```python
from build123d import *

# Parameters (mm, degrees)
F0_R     = 46.99
F0_R_2   = 46.5836
F1_DEPTH = 9.9314
F2_W     = 5.08
F2_H     = 12.7
F3_DEPTH = 76.2
F4_W     = 5.08
F4_H     = 12.7
F5_DEPTH = 76.2


with BuildPart() as f1:
    # F0 (on Top) → F1 (new body)
    with BuildSketch(Plane.XY):
        Circle(F0_R)
        Circle(F0_R_2, mode=Mode.SUBTRACT)
    extrude(amount=F1_DEPTH)

    # F2 (on Right) → F3 (cut, symmetric)
    with BuildSketch(Plane.YZ):
        with Locations((0, 7.4041)):
            Rectangle(F2_W, F2_H)
    extrude(amount=F3_DEPTH, both=True, mode=Mode.SUBTRACT)

    # F4 (on Front) → F5 (cut, symmetric)
    with BuildSketch(Plane.XZ):
        with Locations((0, 7.4041)):
            Rectangle(F4_W, F4_H)
    extrude(amount=F5_DEPTH, both=True, mode=Mode.SUBTRACT)


solid = f1.part
```
The model under review builds one solid part; all positions refer to its coordinate system, in mm. Give positions to 0.01 mm unless a question says otherwise; leave off trailing zeros. Write each loop counter-clockwise with the first axis right and the second up, starting at its lowest first coordinate (ties: lowest second). Pieces come first, ordered by that corner, then holes. Notation, with made-up numbers: M 56,51.25 L 103,51.25 A22 ccw 103,69.25 Z; hole C 26.25,-28.5 d11. An arc over 180 degrees is marked long. Write item = value, one per line. Start each with the question number.
Q1. Clearance check with flat-ended pins moving along their axes: pin 1 (4 mm diameter, centred on x = -8.5, z = 5, fed in from -Y); pin 2 (4 mm diameter, centred on x = -33, z = 4.5, fed in from -Y); pin 3 (0.5 mm diameter, centred on x = 0, y = 47, fed in from +Z). State where each tip first meets the part, or that it passes through.
Q2. Mouldability with a two-part tool opening along X and no side actions: class faces 1 (the face through (44.432, 13.992, 4.896)), 2 (the face through (43.407, -17.997, 4.896)), 3 (the face through (-33.1, 33.1, 9.931)) as released by +X, released by -X, zero draft, split by the parting line, or undercut.
Q3. We need section A-A (y = 0). State the section outline as (x, z) points.
Q4. We need section C-C (z = 2.25). State the section outline as (x, y) points, plus the area to 3 significant figures.
Q5. For line 1 (Y direction, x = 25.5, z = 9); line 2 (X direction, y = 16, z = 8.25); line 3 (Y direction, x = 22, z = 3), list the stretches that pass through material, from the lowest coordinate up.
Result set:
q1.pin_1 = -46.54
q1.pin_2 = -35.31
q1.pin_3 = 1.05
q2.face_1 = undercut
q2.face_2 = split by the parting line
q2.face_3 = zero draft
q3.outline = M -46.99,0 L -46.58,0 L -46.58,1.05 L -46.99,1.05 Z; M 46.58,0 L 46.99,0 L 46.99,1.05 L 46.58,1.05 Z
q4.outline = M -46.92,-2.54 A46.99 ccw -2.54,-46.92 L -2.54,-46.51 A46.58 cw -46.51,-2.54 Z; M -46.92,2.54 L -46.51,2.54 A46.58 cw -2.54,46.51 L -2.54,46.92 A46.99 ccw Z; M 2.54,-46.92 A46.99 ccw 46.92,-2.54 L 46.51,-2.54 A46.58 cw 2.54,-46.51 Z; M 2.54,46.51 A46.58 cw 46.51,2.54 L 46.92,2.54 A46.99 ccw 2.54,46.92 Z
q4.area = 111 mm2
q5.line_1 = -39.47 to -38.98, 38.98 to 39.47
q5.line_2 = -44.18 to -43.75, 43.75 to 44.18
q5.line_3 = -41.52 to -41.06, 41.06 to 41.52
